Read the model definition and answer for the solid it produces. Units are mm, in the model's axes. Face numbers are marked on the shaded views. A direction names the side the tool comes from. Give positions to 0.01 mm unless a question says otherwise; leave off trailing zeros. Write each loop counter-clockwise with the first axis right and the second up, starting at its lowest first coordinate (ties: lowest second). Pieces come first, ordered by that corner, then holes. Notation, with made-up numbers: (64, -10) -> (87, -10) arc R15 ccw to (87, 3) -> close; hole circle Ø10 at (-1.5, 2.25). An arc over 180 degrees is marked (long way). Write item = value, one per line.
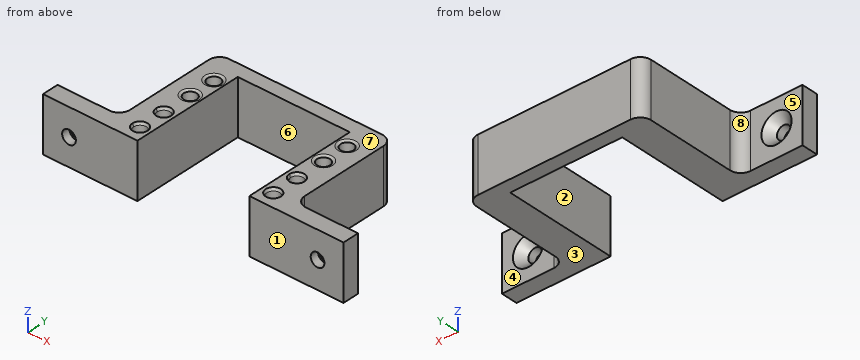
from build123d import *

# Parameters (mm, degrees)
SKETCH1_W             = 18.495
SKETCH1_H             = 20.8
SKETCH1_W_2           = 10
SKETCH1_W_3           = 37.395
BOSS_EXTRUDE1_DEPTH   = 20
SKETCH6_W             = 106.79
SKETCH6_H             = 20
BOSS_EXTRUDE4_DEPTH   = 5
SKETCH9_R             = 2.35
CUT_EXTRUDE1_DEPTH    = 10
SKETCH10_W            = 20
SKETCH10_H            = 25.8
CUT_EXTRUDE2_DEPTH    = 17
SKETCH11_W            = 20
SKETCH11_H            = 25.8
CUT_EXTRUDE3_DEPTH    = 26
CHAMFER1_SIZE         = 1
CHAMFER1_SIZE2        = 0.424474816
MIRROR1_2_OUTLINE_R   = 2.35
MIRROR1_2_OUTLINE_R_2 = 2.774474816
MIRROR1_2_DEPTH       = 20
MIRROR1_3_OUTLINE_R   = 2.35
MIRROR1_3_OUTLINE_R_2 = 2.774474816
MIRROR1_3_DEPTH       = 10
SKETCH12_W            = 63.79
SKETCH12_H            = 20
CUT_EXTRUDE4_DEPTH    = 5
SKETCH13_W            = 20
SKETCH13_H            = 6
BOSS_EXTRUDE5_DEPTH   = 23
FILLET2_R             = 4
SKETCH14_R            = 2.5
CUT_EXTRUDE5_DEPTH    = 6
CHAMFER2_SIZE         = 3


with BuildPart() as part:
    # Sketch1 → Boss-Extrude1 (new body)
    with BuildSketch(Plane.XY):
        with Locations((-39.1475, 0)):
            Rectangle(SKETCH1_W, SKETCH1_H)
        with Locations((-53.395, 0)):
            Rectangle(SKETCH1_W_2, SKETCH1_H)
        with Locations((29.6975, 0)):
            Rectangle(SKETCH1_W_3, SKETCH1_H)
    extrude(amount=BOSS_EXTRUDE1_DEPTH)

    # Sketch6 → Boss-Extrude4 (add)
    with BuildSketch(Plane(origin=(0, 10.4, 0), x_dir=(1, 0, 0), z_dir=(0, 1, 0))):
        with Locations((-5, -10)):
            Rectangle(SKETCH6_W, SKETCH6_H)
    extrude(amount=BOSS_EXTRUDE4_DEPTH)

    # Sketch9 → Cut-Extrude1 (cut)
    with BuildSketch(Plane.XY.offset(20)):
        with Locations((14.89, -4.9)):
            Circle(SKETCH9_R)
        with Locations(Location((14.89, 4.9, 0), (0, 0, 180))):
            Circle(SKETCH9_R)
        with Locations(Location((-33.79, -4.9, 0), (0, 0, 180))):
            Circle(SKETCH9_R)
        with Locations((-33.79, 4.9)):
            Circle(SKETCH9_R)
    extrude(amount=-CUT_EXTRUDE1_DEPTH, mode=Mode.SUBTRACT)

    # Sketch10 → Cut-Extrude2 (cut)
    with BuildSketch(Plane.ZY.offset(58.395)):
        with Locations((10, 2.5)):
            Rectangle(SKETCH10_W, SKETCH10_H)
    extrude(amount=-CUT_EXTRUDE2_DEPTH, mode=Mode.SUBTRACT)

    # Sketch11 → Cut-Extrude3 (cut)
    with BuildSketch(Plane(origin=(48.395, 0, 0), x_dir=(0, 0, -1), z_dir=(1, 0, 0))):
        with Locations((-10, 2.5)):
            Rectangle(SKETCH11_W, SKETCH11_H)
    extrude(amount=-CUT_EXTRUDE3_DEPTH, mode=Mode.SUBTRACT)

    # Chamfer1
    chamfer1_edges = [part.edges().sort_by_distance(p)[0] for p in [
        (17.24, 4.9, 20),
        (-31.44, -4.9, 20),
        (-36.14, 4.9, 20),
        (12.54, -4.9, 20),
    ]]
    chamfer1_side = [part.faces().sort_by_distance(p)[0] for p in [
        (-35.6475, -9.711900872, 20),
    ]]
    chamfer(chamfer1_edges, length=CHAMFER1_SIZE, length2=CHAMFER1_SIZE2, reference=chamfer1_side[0])



with BuildPart() as body_2:
    # Mirror1: read off the stored shape, not the designer's step
    # Mirror1 outline → Mirror1 (revolve)
    with BuildSketch(Plane(origin=(14.89, -25.7, 0), x_dir=(1, 0, 0), z_dir=(0, -1, 0))):
        Polygon((2.35, 19), (2.35, 10), (2.774474816, 10), (2.774474816, 20), align=None)
    revolve(axis=Axis((14.89, -25.7, 0), (0, 0, 1)))


with BuildPart() as part_1:
    add(part.part)

    add(body_2.part)  # Mirror1 2 merges body 2
    # Mirror1 2 outline → Mirror1 2 (add)
    with BuildSketch(Plane.XY):
        Polygon((-41.395, -10.4), (-41.395, -36.2), (22.395, -36.2), (22.395, -10.4), (11, -10.4), (11, -31.2), (-29.9, -31.2), (-29.9, -10.4), align=None)
        with Locations((-33.79, -25.7)):
            Circle(MIRROR1_2_OUTLINE_R, mode=Mode.SUBTRACT)
        with Locations((14.89, -25.7)):
            Circle(MIRROR1_2_OUTLINE_R_2, mode=Mode.SUBTRACT)
        with Locations((-33.79, -15.9)):
            Circle(MIRROR1_2_OUTLINE_R, mode=Mode.SUBTRACT)
        with Locations((14.89, -15.9)):
            Circle(MIRROR1_2_OUTLINE_R, mode=Mode.SUBTRACT)
    extrude(amount=MIRROR1_2_DEPTH)

    # Mirror1 3 outline → Mirror1 3 (add)
    with BuildSketch(Plane.XY):
        with Locations((14.89, -15.9)):
            Circle(MIRROR1_3_OUTLINE_R)
        with Locations((-33.79, -25.7)):
            Circle(MIRROR1_3_OUTLINE_R)
        with Locations((-33.79, -15.9)):
            Circle(MIRROR1_3_OUTLINE_R)
        with Locations((14.89, -25.7)):
            Circle(MIRROR1_3_OUTLINE_R_2)
    extrude(amount=MIRROR1_3_DEPTH)

    # Mirror1 4: loft between two sections, ruled curve by curve
    mirror1_4_from = [
        Edge.make_three_point_arc((17.24, -15.9, 19), (14.89, -13.55, 19), (12.54, -15.9, 19)),
        Edge.make_three_point_arc((12.54, -15.9, 19), (14.89, -18.25, 19), (17.24, -15.9, 19)),
    ]
    mirror1_4_to = [
        Edge.make_three_point_arc((17.664474816, -15.9, 20), (14.89, -13.125525184, 20), (12.115525184, -15.9, 20)),
        Edge.make_three_point_arc((12.115525184, -15.9, 20), (14.89, -18.674474816, 20), (17.664474816, -15.9, 20)),
    ]
    mirror1_4 = Solid(Shell([*[Face.make_surface_from_curves(mirror1_4_from[k], mirror1_4_to[k]) for k in range(2)], Face(Wire(mirror1_4_from)), Face(Wire(mirror1_4_to))]))
    add(mirror1_4, mode=Mode.SUBTRACT)

    # Mirror1 5: loft between two sections, ruled curve by curve
    mirror1_5_from = [
        Edge.make_three_point_arc((-31.44, -25.7, 19), (-33.79, -23.35, 19), (-36.14, -25.7, 19)),
        Edge.make_three_point_arc((-36.14, -25.7, 19), (-33.79, -28.05, 19), (-31.44, -25.7, 19)),
    ]
    mirror1_5_to = [
        Edge.make_three_point_arc((-31.015525184, -25.7, 20), (-33.79, -22.925525184, 20), (-36.564474816, -25.7, 20)),
        Edge.make_three_point_arc((-36.564474816, -25.7, 20), (-33.79, -28.474474816, 20), (-31.015525184, -25.7, 20)),
    ]
    mirror1_5 = Solid(Shell([*[Face.make_surface_from_curves(mirror1_5_from[k], mirror1_5_to[k]) for k in range(2)], Face(Wire(mirror1_5_from)), Face(Wire(mirror1_5_to))]))
    add(mirror1_5, mode=Mode.SUBTRACT)

    # Mirror1 6: loft between two sections, ruled curve by curve
    mirror1_6_from = [
        Edge.make_three_point_arc((-31.44, -15.9, 19), (-33.79, -13.55, 19), (-36.14, -15.9, 19)),
        Edge.make_three_point_arc((-36.14, -15.9, 19), (-33.79, -18.25, 19), (-31.44, -15.9, 19)),
    ]
    mirror1_6_to = [
        Edge.make_three_point_arc((-31.015525184, -15.9, 20), (-33.79, -13.125525184, 20), (-36.564474816, -15.9, 20)),
        Edge.make_three_point_arc((-36.564474816, -15.9, 20), (-33.79, -18.674474816, 20), (-31.015525184, -15.9, 20)),
    ]
    mirror1_6 = Solid(Shell([*[Face.make_surface_from_curves(mirror1_6_from[k], mirror1_6_to[k]) for k in range(2)], Face(Wire(mirror1_6_from)), Face(Wire(mirror1_6_to))]))
    add(mirror1_6, mode=Mode.SUBTRACT)

    # Sketch12 → Cut-Extrude4 (cut)
    with BuildSketch(Plane(origin=(0, -36.2, 0), x_dir=(-1, 0, 0), z_dir=(0, -1, 0))):
        with Locations((9.5, -10)):
            Rectangle(SKETCH12_W, SKETCH12_H)
    extrude(amount=-CUT_EXTRUDE4_DEPTH, mode=Mode.SUBTRACT)

    # Sketch13 → Boss-Extrude5 (add)
    with BuildSketch(Plane(origin=(22.395, 0, 0), x_dir=(0, 0, -1), z_dir=(1, 0, 0))):
        with Locations((-10, -28.2)):
            Rectangle(SKETCH13_W, SKETCH13_H)
    boss_extrude5 = extrude(amount=BOSS_EXTRUDE5_DEPTH)

    # Mirror2: Boss-Extrude5 across plane
    add(boss_extrude5.mirror(Plane(origin=(-9.5, 0, 0), x_dir=(0, 0, 1), z_dir=(1, 0, 0))))

    # Fillet2
    fillet2_edges = [part_1.edges().sort_by_distance(p)[0] for p in [
        (22.395, -25.2, 10),
        (-41.395, -25.2, 10),
        (-41.395, 15.4, 10),
        (22.395, 15.4, 10),
    ]]
    fillet(fillet2_edges, radius=FILLET2_R)

    # Sketch14 → Cut-Extrude5 (cut)
    with BuildSketch(Plane(origin=(0, -25.2, 0), x_dir=(1, 0, 0), z_dir=(0, 1, 0))):
        with Locations(Location((35.895, -10, 0), (0, 0, 270))):
            Circle(SKETCH14_R)
    cut_extrude5 = extrude(amount=-CUT_EXTRUDE5_DEPTH, mode=Mode.SUBTRACT)

    # Mirror5: Cut-Extrude5 across plane
    add(cut_extrude5.mirror(Plane(origin=(-9.5, 0, 0), x_dir=(0, 0, 1), z_dir=(1, 0, 0))), mode=Mode.SUBTRACT)

    # Chamfer2
    chamfer2_edges = [part_1.edges().sort_by_distance(p)[0] for p in [
        (35.895, -25.2, 7.5),
        (-54.895, -25.2, 7.5),
    ]]
    chamfer(chamfer2_edges, length=CHAMFER2_SIZE)


solid = part_1.part
(1) Given P1, Ø10, axis at y = -9.5, z = 9, coming from the -X side (3 decimals); P2, Ø4, axis at x = -33.79, y = -4.9, coming from the +Z side; P3, Ø10, axis at y = -5.5, z = 14, coming from the +X side (3 decimals), each flat-ended and moving along its own axis, determine where each tip first touches the part or whether it passes through.
Checks:
P1 = -41.395
P2 = 10
P3 = 22.395
(2) The part is cut by section C-C on x = -22.5. Determine the outline of the cut face in (y, z), plus the area to 3 significant figures.
Checks:
outline = (10.4, 0) -> (15.4, 0) -> (15.4, 20) -> (10.4, 20) -> close
area = 100 mm²
(3) The part is cut by section A-A on z = 16.5. Count the separate pieces of the cut face and the enclosed holes in it, plus the area to 3 significant figures.
Checks:
separate_pieces = 1
enclosed_holes = 8
area = 1,410 mm²
(4) The part is cut by section B-B on y = -4.9. Determine the outline of the cut face in (x, z) (3 decimals).
Checks:
outline = (-41.395, 0) -> (-29.9, 0) -> (-29.9, 20) -> (-30.44, 20) -> (-31.44, 19.576) -> (-31.44, 10) -> (-36.14, 10) -> (-36.14, 19.576) -> (-37.14, 20) -> (-41.395, 20) -> close; (11, 0) -> (22.395, 0) -> (22.395, 20) -> (18.24, 20) -> (17.24, 19.576) -> (17.24, 10) -> (12.54, 10) -> (12.54, 19.576) -> (11.54, 20) -> (11, 20) -> close
(5) For a pull along X with two mould halves and no side action, classify the marked faces 6, 7 and 8 as released by +X, released by -X, zero draft, split by the parting line, or undercut.
Checks:
face_6 = undercut
face_7 = zero draft
face_8 = released by -X
(6) A tool of negligible diameter and unlimited length cuts with its end or side. For the marked faces 1, 2, 3, 4 and 5, from which of +Z, -Z, +X, -X, +Y, -Y can it reach the whole face along a straight path? Write none if from no direction.
Checks:
face_1 = +Z, -Z, +X, -X, -Y
face_2 = +Z, -Z, -Y
face_3 = -Z, +X, -X, +Y, -Y
face_4 = +Z, -Z, +X, +Y
face_5 = +Z, -Z, -X, +Y
(7) Consider L1, parallel to Y at x = 14.89, z = 14; L2, parallel to X at y = -21.5, z = 3.5; L3, parallel to X at y = -15.9, z = 17.25 (3 decimals). Determine where each line is inside the solid, lowest interval first.
Checks:
L1 = -31.2 to -28.05, -23.35 to -18.25, -13.55 to -7.25, -2.55 to 2.55, 7.25 to 15.4
L2 = -41.41 to -29.9, 11 to 22.41
L3 = -41.395 to -36.14, -31.44 to -29.9, 11 to 12.54, 17.24 to 22.395
